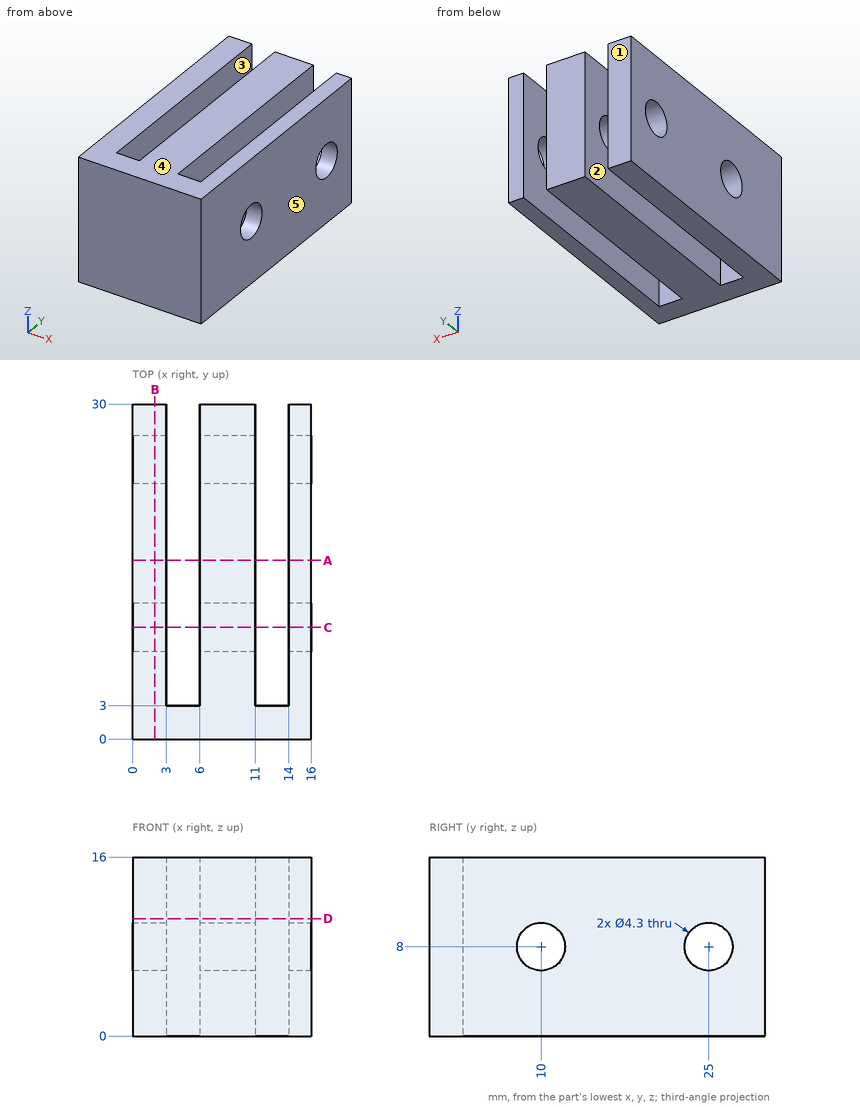
Can you work these out from the drawing? Everything is in mm from the part's minimum corner. A direction names the side the tool comes from. Give positions to 0.01 mm unless a question says otherwise; leave off trailing zeros. Loops run counter-clockwise (first coordinate to the right, second up) from the corner with the lowest first, then second, coordinate; pieces in that order, holes last. Notation, with made-up numbers: M 52,85 L 65,85 A24 ccw 65,115 Z; hole C -20.5,75 d5. An arc over 180 degrees is marked long. Put each result on its own line as item: value. Start each with the question number.
(1) If we mould it in two halves opening along X, with no side actions, what happens to the marked faces 3, 4 and 5? For each: +X half, -X half, draft (parallel to the pull), parting line (faces both ways), or undercut.
(2) I want a section at B-B on x = 2. Please give me the cut outline in (y, z), then the cut area to 3 significant figures.
(3) For the marked faces 1 and 2, which set-ups out of +Z, -Z, +X, -X, +Y, -Y let a thin tool reach every point of the face, with its end or its side?
(4) I want a section at C-C on y = 10. Please give me the cut outline in (x, z), then the cut area to 3 significant figures.
(5) I want a section at D-D on z = 10.5. Please give me the cut outline in (x, y).
(6) Will these pins go through, and if not, where does the flat tip stop? pin 1 Ø1.5 at (x, z) = (4.5, 5) entering from +Y; pin 2 Ø4 at (y, z) = (25, 8) entering from -X.
(7) I want a section at A-A on y = 16. Please give me the cut outline in (x, z).
(8) I need wall thicknesses on line 1 along Y through (x, z) = (2.3, 8); line 2 along X through (y, z) = (4.75, 6.5); line 3 along Y through (x, z) = (2.5, 6.25). Which ranges of each line are inside material? Lowest first, please. Write a range as [from, to].
Answer block:
1. face 3: undercut
1. face 4: draft
1. face 5: +X half
2. outline: M 0,0 L 30,0 L 30,16 L 0,16 Z; hole C 10,8 d4.3; hole C 25,8 d4.3
2. area: 451 mm^2
3. face 1: +Z, -Z, +X, -X, +Y
3. face 2: +Z, -Z, +Y
4. outline: M 0,0 L 3,0 L 3,5.85 L 0,5.85 Z; M 0,10.15 L 3,10.15 L 3,16 L 0,16 Z; M 6,0 L 11,0 L 11,5.85 L 6,5.85 Z; M 6,10.15 L 11,10.15 L 11,16 L 6,16 Z; M 14,0 L 16,0 L 16,5.85 L 14,5.85 Z; M 14,10.15 L 16,10.15 L 16,16 L 14,16 Z
4. area: 117 mm^2
5. outline: M 0,0 L 16,0 L 16,30 L 14,30 L 14,3 L 11,3 L 11,30 L 6,30 L 6,3 L 3,3 L 3,30 L 0,30 Z
6. pin 1: y = 3
6. pin 2: through
7. outline: M 0,0 L 3,0 L 3,16 L 0,16 Z; M 6,0 L 11,0 L 11,16 L 6,16 Z; M 14,0 L 16,0 L 16,16 L 14,16 Z
8. line 1: [0, 7.85], [12.15, 22.85], [27.15, 30]
8. line 2: [0, 3], [6, 11], [14, 16]
8. line 3: [0, 8.75], [11.25, 23.75], [26.25, 30]
